```python
from build123d import *

# Parameters (mm, degrees)
F0_W     = 136.31
F0_H     = 16.17
F1_DEPTH = 88.79
F3_DEPTH = 88.79
F5_DEPTH = 88.79
F6_R     = 5
F8_D     = 16.17


with BuildPart() as f1:
    # F0 (on Front) → F1 (new body)
    with BuildSketch(Plane.XZ):
        with Locations((0, 8.085)):
            Rectangle(F0_W, F0_H)
    extrude(amount=-F1_DEPTH)

    # F2 (on face) → F3 (join)
    with BuildSketch(Plane.XZ):
        Polygon((-15, 16.17), (0, 16.17), (15, 16.17), (11.445, 19.725), (-11.445, 19.725), align=None)
    extrude(amount=-F3_DEPTH)

    # F4 (on Front) → F5 (cut)
    with BuildSketch(Plane.XZ):
        Polygon((-15, 0), (0, 0), (15, 0), (11.4644660941, 3.5355339059), (-11.4644660941, 3.5355339059), align=None)
    extrude(amount=-F5_DEPTH, mode=Mode.SUBTRACT)

    # F6
    f6_edges = [f1.edges().sort_by_distance(p)[0] for p in [
        (68.155, 88.79, 8.085),
        (-68.155, 88.79, 8.085),
        (68.155, 0, 8.085),
        (-68.155, 0, 8.085),
    ]]
    fillet(f6_edges, radius=F6_R)

    # F8 (through all)
    with Locations(Plane(origin=(0, 0, 0), x_dir=(1, 0, 0), z_dir=(0, 0, -1))):
        with Locations((-50.155, -71), (-50.155, -16), (49.845, -71), (49.845, -16)):
            Hole(F8_D / 2)


solid = f1.part
```
Geometry check sheet. Reference: the model listing, model coordinates, mm. A direction names the side the tool comes from. Coordinates: 2 decimals unless noted, no trailing zeros. Loops run counter-clockwise (first coordinate to the right, second up) from the corner with the lowest first, then second, coordinate; pieces in that order, holes last.
Item 1: Go/stop test with flat-tipped pins: pin 1 Ø16 at (x, y) = (-38.5, 29.5) entering from +Z; pin 2 Ø6 at (x, y) = (32, 53.5) entering from -Z; pin 3 Ø25 at (x, y) = (-0.5, 49.5) entering from -Z. Record where each tip stops, or that it passes through.
Item 2: Thickness scan on line 1 (X direction, y = 71, z = 8) (3 decimals); line 2 (X direction, y = 68.5, z = 3) (3 decimals); line 3 (Y direction, x = -44.5, z = 12.25). Record the ranges inside material, lowest first.
Item 3: Sectioned sample at A-A, the plane y = 16. Record the boundary of the cut face in (x, z) (3 decimals).
Item 4: Sectioned sample at C-C, the plane x = 43.5. Record the boundary of the cut face in (y, z).
Item 5: Access from +Z, -Z, +X, -X, +Y, -Y to the whole of each face (thin tool, end or side, straight path). Record for faces 1 (the face through (-13.2, 43.77, 17.97)), 2 (the face through (41, 44, 16.17)), 3 (the face through (-13, 44, 2)).
Item 6: Sectioned sample at D-D, the plane y = 49. Record the boundary of the cut face in (x, z) (3 decimals), then the cut area to 3 significant figures.
Item 7: Sectioned sample at B-B, the plane z = 11.5. Record the boundary of the cut face in (x, y) (3 decimals).
Item 8: Release check for a two-part mould opening along X. For faces 4 (the face through (66.651, 87.364, 8.198)), 5 (the face through (-68.155, 44, 8)), 6 (the face through (-1, 0, 8)), 7 (the face through (57.92, 15.64, 8.2)) record: released by +X, released by -X, zero draft, split by the parting line, or undercut.
Check result:
1. pin 1: stops at z = 16.17
1. pin 2: stops at z = 0
1. pin 3: stops at z = 2
2. line 1: x = -68.155 to -58.24, -42.07 to 41.76, 57.93 to 68.155
2. line 2: x = -68.155 to -57.844, -42.466 to -12, 12 to 42.156, 57.534 to 68.155
2. line 3: y = 0 to 10.22, 21.78 to 65.22, 76.78 to 88.79
3. outline: (-68.155, 0) - (-58.24, 0) - (-58.24, 16.17) - (-68.155, 16.17) - close; (-42.07, 0) - (-15, 0) - (-11.464, 3.536) - (11.464, 3.536) - (15, 0) - (41.76, 0) - (41.76, 16.17) - (15, 16.17) - (11.445, 19.725) - (-11.445, 19.725) - (-15, 16.17) - (-42.07, 16.17) - close; (57.93, 0) - (68.155, 0) - (68.155, 16.17) - (57.93, 16.17) - close
4. outline: (0, 0) - (10.99, 0) - (10.99, 16.17) - (0, 16.17) - close; (21.01, 0) - (65.99, 0) - (65.99, 16.17) - (21.01, 16.17) - close; (76.01, 0) - (88.79, 0) - (88.79, 16.17) - (76.01, 16.17) - close
5. face 1: +Z, -X, +Y, -Y
5. face 2: +Z, +X, +Y, -Y
5. face 3: -Z, +Y, -Y
6. outline: (-68.155, 0) - (-15, 0) - (-11.464, 3.536) - (11.464, 3.536) - (15, 0) - (68.155, 0) - (68.155, 16.17) - (15, 16.17) - (11.445, 19.725) - (-11.445, 19.725) - (-15, 16.17) - (-68.155, 16.17) - close
6. area: 2,200 mm2
7. outline: (-68.155, 5) arc R5 ccw to (-63.155, 0) - (63.155, 0) arc R5 ccw to (68.155, 5) - (68.155, 83.79) arc R5 ccw to (63.155, 88.79) - (-63.155, 88.79) arc R5 ccw to (-68.155, 83.79) - close; hole circle Ø16.17 at (-50.155, 16); hole circle Ø16.17 at (-50.155, 71); hole circle Ø16.17 at (49.845, 16); hole circle Ø16.17 at (49.845, 71)
8. face 4: released by +X
8. face 5: released by -X
8. face 6: zero draft
8. face 7: undercut
